Input: part model. Units: mm. Frame: model coordinates. Face numbers are marked on the shaded views. A direction names the side the tool comes from. Give positions to 0.01 mm unless a question says otherwise; leave off trailing zeros. Write each loop counter-clockwise with the first axis right and the second up, starting at its lowest first coordinate (ties: lowest second). Pieces come first, ordered by that corner, then holes. Notation, with made-up numbers: (18.25, -36.75) -> (36.25, -36.75) arc R27 cw to (36.25, -9.75) -> close; hole circle Ø5 at (70.25, 59). An arc over 180 degrees is marked (long way). Return JSON: item names as keys, results as strings. Group by question number.
Item 1: Section C-C, the plane z = 1.5. Return loops of the section in (x, y).
Item 2: Line query: line 1 (Z direction, x = -0.6, y = -0.2); line 2 (Z direction, x = 1.75, y = 0.35); line 3 (X direction, y = -0.05, z = 4). Output: solid intervals per line, ascending. Write a range as [from, to].
Item 3: Mould query, pull axis Y, two halves, no side actions, for the marked faces 3 and 4. Classes: released by +Y, released by -Y, zero draft, split by the parting line, or undercut.
Item 4: Section B-B, the plane y = 0. Return loops of the section in (x, z).
Item 5: Section A-A, the plane x = 0. Return loops of the section in (y, z), then the cut area to 3 significant figures.
Item 6: Pin query (flat end, axial travel): P1, Ø0.6, axis at x = -1, z = 0, coming from the +Y side; P2, Ø2, axis at x = 0.5, z = 4.5, coming from the +Y side. Return the tip coordinate at first contact, or that it passes through.
Item 7: Section D-D, the plane x = 1.65. Return loops of the section in (y, z), then the cut area to 3 significant figures.
Item 8: Set-up query: the marked faces 1 and 2. Return all of +Z, -Z, +X, -X, +Y, -Y with unobstructed straight access to the full face (end or side cutting, diameter ignored); none if empty.
from build123d import *

# Parameters (mm, degrees)
ESQUISSE1_R             = 2
BOSS_EXTRU_1_DEPTH      = 2
ESQUISSE2_R             = 1.3
BOSS_EXTRU_2_DEPTH      = 7.5
ESQUISSE3_W             = 5.055349602
ESQUISSE3_H             = 0.46857679
ENL_V_MAT_EXTRU_1_DEPTH = 0.5


with BuildPart() as part:
    # Esquisse1 → Boss.-Extru.1 (new body)
    with BuildSketch(Plane.XY):
        Circle(ESQUISSE1_R)
    extrude(amount=BOSS_EXTRU_1_DEPTH)

    # Esquisse2 → Boss.-Extru.2 (add)
    with BuildSketch(Plane.XY.offset(2)):
        Circle(ESQUISSE2_R)
    extrude(amount=BOSS_EXTRU_2_DEPTH)

    # Esquisse3 → Enlèv. mat.-Extru.1 (cut)
    with BuildSketch(Plane(origin=(0, 0, 0), x_dir=(-1, 0, 0), z_dir=(0, 0, -1))):
        Rectangle(ESQUISSE3_W, ESQUISSE3_H)
    extrude(amount=-ENL_V_MAT_EXTRU_1_DEPTH, mode=Mode.SUBTRACT)


solid = part.part
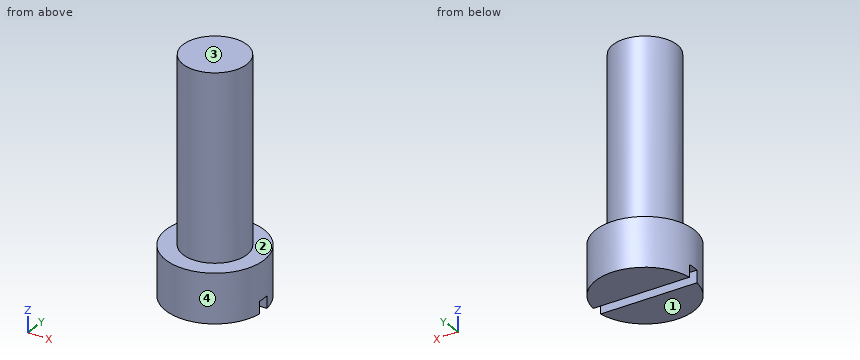
Answer below:
{
 "1": {"outline": "circle Ø4 at (0, 0)"},
 "2": {"line 1": "z = [0.5, 9.5]", "line 2": "z = [0, 2]", "line 3": "x = [-1.3, 1.3]"},
 "3": {"face 3": "zero draft", "face 4": "split by the parting line"},
 "4": {"outline": "(-2, 0.5) -> (2, 0.5) -> (2, 2) -> (1.3, 2) -> (1.3, 9.5) -> (-1.3, 9.5) -> (-1.3, 2) -> (-2, 2) -> close"},
 "5": {"outline": "(-2, 0) -> (-0.23, 0) -> (-0.23, 0.5) -> (0.23, 0.5) -> (0.23, 0) -> (2, 0) -> (2, 2) -> (1.3, 2) -> (1.3, 9.5) -> (-1.3, 9.5) -> (-1.3, 2) -> (-2, 2) -> close", "area": "27.3 mm2"},
 "6": {"P1": "stops at y = 1.87", "P2": "stops at y = 1.3"},
 "7": {"outline": "(-1.13, 0) -> (-0.23, 0) -> (-0.23, 0.5) -> (0.23, 0.5) -> (0.23, 0) -> (1.13, 0) -> (1.13, 2) -> (-1.13, 2) -> close", "area": "4.29 mm2"},
 "8": {"face 1": "-Z, +X, -X, +Y, -Y", "face 2": "+Z"}
}
